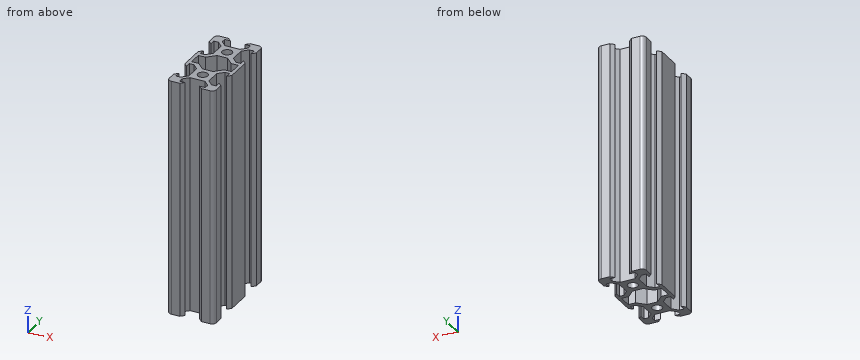
from build123d import *

# Parameters (mm, degrees)
SKETCH001_R = 2.1
PAD_DEPTH   = 100


with BuildPart() as part:
    # Sketch001 → Pad (new body)
    with BuildSketch(Plane.XY):
        with BuildLine():
            Line((10, 0), (10, -5.42))
            Line((10, -5.42), (8.545, -6.875))
            Line((8.545, -6.875), (8.545, -4.5))
            Line((8.545, -4.5), (6.56066, -4.5))
            Line((6.56066, -4.5), (4.245, -6.81566))
            Line((4.245, -6.81566), (4.245, -13.18434))
            Line((4.245, -13.18434), (6.56066, -15.5))
            Line((6.56066, -15.5), (8.545, -15.5))
            Line((8.545, -15.5), (8.545, -13.125))
            Line((8.545, -13.125), (10, -14.58))
            Line((10, -14.58), (10, -18.2))
            ThreePointArc((8.2, -20), (9.472792, -19.472792), (10, -18.2))
            Line((8.2, -20), (4.58, -20))
            Line((4.58, -20), (3.125, -18.545))
            Line((3.125, -18.545), (5.5, -18.545))
            Line((5.5, -18.545), (5.5, -16.56066))
            Line((5.5, -16.56066), (3.18434, -14.245))
            Line((3.18434, -14.245), (-3.18434, -14.245))
            Line((-3.18434, -14.245), (-5.5, -16.56066))
            Line((-5.5, -16.56066), (-5.5, -18.545))
            Line((-5.5, -18.545), (-3.125, -18.545))
            Line((-3.125, -18.545), (-4.58, -20))
            Line((-4.58, -20), (-8.2, -20))
            ThreePointArc((-10, -18.2), (-9.472792, -19.472792), (-8.2, -20))
            Line((-10, -18.2), (-10, -14.58))
            Line((-10, -14.58), (-8.545, -13.125))
            Line((-8.545, -13.125), (-8.545, -15.5))
            Line((-8.545, -15.5), (-6.56066, -15.5))
            Line((-6.56066, -15.5), (-4.245, -13.18434))
            Line((-4.245, -13.18434), (-4.245, -6.81566))
            Line((-4.245, -6.81566), (-6.56066, -4.5))
            Line((-6.56066, -4.5), (-8.545, -4.5))
            Line((-8.545, -4.5), (-8.545, -6.875))
            Line((-8.545, -6.875), (-10, -5.42))
            Line((-10, -5.42), (-10, 0))
            Line((-10, 5.42), (-10, 0))
            Line((-8.545, 6.875), (-10, 5.42))
            Line((-8.545, 4.5), (-8.545, 6.875))
            Line((-6.56066, 4.5), (-8.545, 4.5))
            Line((-4.245, 6.81566), (-6.56066, 4.5))
            Line((-4.245, 13.18434), (-4.245, 6.81566))
            Line((-6.56066, 15.5), (-4.245, 13.18434))
            Line((-8.545, 15.5), (-6.56066, 15.5))
            Line((-8.545, 13.125), (-8.545, 15.5))
            Line((-10, 14.58), (-8.545, 13.125))
            Line((-10, 18.2), (-10, 14.58))
            ThreePointArc((-8.2, 20), (-9.472792, 19.472792), (-10, 18.2))
            Line((-4.58, 20), (-8.2, 20))
            Line((-3.125, 18.545), (-4.58, 20))
            Line((-5.5, 18.545), (-3.125, 18.545))
            Line((-5.5, 16.56066), (-5.5, 18.545))
            Line((-3.18434, 14.245), (-5.5, 16.56066))
            Line((3.18434, 14.245), (-3.18434, 14.245))
            Line((5.5, 16.56066), (3.18434, 14.245))
            Line((5.5, 18.545), (5.5, 16.56066))
            Line((3.125, 18.545), (5.5, 18.545))
            Line((4.58, 20), (3.125, 18.545))
            Line((8.2, 20), (4.58, 20))
            ThreePointArc((10, 18.2), (9.472792, 19.472792), (8.2, 20))
            Line((10, 14.58), (10, 18.2))
            Line((8.545, 13.125), (10, 14.58))
            Line((8.545, 15.5), (8.545, 13.125))
            Line((6.56066, 15.5), (8.545, 15.5))
            Line((4.245, 13.18434), (6.56066, 15.5))
            Line((4.245, 6.81566), (4.245, 13.18434))
            Line((6.56066, 4.5), (4.245, 6.81566))
            Line((8.545, 4.5), (6.56066, 4.5))
            Line((8.545, 6.875), (8.545, 4.5))
            Line((10, 5.42), (8.545, 6.875))
            Line((10, 0), (10, 5.42))
        make_face()
        with Locations((0, -10)):
            Circle(SKETCH001_R, mode=Mode.SUBTRACT)
        with Locations((0, 10)):
            Circle(SKETCH001_R, mode=Mode.SUBTRACT)
        Polygon((-8.545, 0), (-8.545, -2.788399), (-5.427946, -2.788399), (-2.248662, -5.967683), (2.248662, -5.967683), (5.427946, -2.788399), (8.545, -2.788399), (8.545, 0), (8.545, 2.788399), (5.427946, 2.788399), (2.248662, 5.967683), (-2.248662, 5.967683), (-5.427946, 2.788399), (-8.545, 2.788399), align=None, mode=Mode.SUBTRACT)
    extrude(amount=PAD_DEPTH)


solid = part.part
Build history of the part. All positions in model axes, mm. Coordinates: 2 decimals unless noted, no trailing zeros. Write each loop counter-clockwise with the first axis right and the second up, starting at its lowest first coordinate (ties: lowest second). Pieces come first, ordered by that corner, then holes.
(1) Cut at C-C on z = 52.5. State how many separate pieces and enclosed holes the cut face has, and give its area (4 significant figures).
(2) Cut at D-D on y = -1.5. List the corners of the cut face in (x, z) (3 decimals), and give its area (3 significant figures).
(3) Cut at B-B on x = 0. List the corners of the cut face in (y, z) (3 decimals).
(4) Pin check, flat tips, straight feed: pin 1 Ø7 at (y, z) = (-10.5, 40.5) entering from +X; pin 2 Ø5 at (x, z) = (0, 60.5) entering from -Y (3 decimals); pin 3 Ø1 at (x, z) = (-0.5, 85.5) entering from +Y (3 decimals). Stop position of each tip, or through.
(5) Drill centre lines: line 1 (Y direction, x = 0, z = 37) (3 decimals); line 2 (Y direction, x = 8, z = 78); line 3 (X direction, y = 5, z = 42.5) (3 decimals). Where is each one in solid material? Low to high.
(6) Cut at A-A on y = 10. List the corners of the cut face in (x, z) (3 decimals).
Working result:
1. separate pieces: 1
1. enclosed holes: 3
1. area: 306.5 mm2
2. outline: (-10, 0) - (-8.545, 0) - (-8.545, 100) - (-10, 100) - close; (8.545, 0) - (10, 0) - (10, 100) - (8.545, 100) - close
2. area: 291 mm2
3. outline: (-14.245, 0) - (-12.1, 0) - (-12.1, 100) - (-14.245, 100) - close; (-7.9, 0) - (-5.968, 0) - (-5.968, 100) - (-7.9, 100) - close; (5.968, 0) - (7.9, 0) - (7.9, 100) - (5.968, 100) - close; (12.1, 0) - (14.245, 0) - (14.245, 100) - (12.1, 100) - close
4. pin 1: stops at x = 9.42
4. pin 2: stops at y = -14.245
4. pin 3: stops at y = 14.245
5. line 1: y = -14.245 to -12.1, -7.9 to -5.968, 5.968 to 7.9, 12.1 to 14.245
5. line 2: y = -20 to -15.5, -4.5 to -2.79, 2.79 to 4.5, 15.5 to 20
5. line 3: x = -10 to -8.545, -6.061 to -3.216, 3.216 to 6.061, 8.545 to 10
6. outline: (-4.245, 0) - (-2.1, 0) - (-2.1, 100) - (-4.245, 100) - close; (2.1, 0) - (4.245, 0) - (4.245, 100) - (2.1, 100) - close
